Check sheet for the modelled part. Datum: model origin and axes. Units: mm. Round coordinates to 2 decimals unless told otherwise and drop trailing zeros. Loops run counter-clockwise (first coordinate to the right, second up) from the corner with the lowest first, then second, coordinate; pieces in that order, holes last. Notation, with made-up numbers: (5.5, 74) -> (42.5, 74) arc R19 cw to (42.5, 83) -> close; hole circle Ø2 at (71.5, 35). An arc over 180 degrees is marked (long way). Use one line per item in the form item = value. Start each with the question number.
(1) Sectioned sample at B-B (x = 4.75). Record the cut outline in (y, z), and give its area (3 significant figures).
(2) Material ranges on probe 1 along X at (y, z) = (40.5, -6.75); probe 2 along Y at (x, z) = (8.25, -12); probe 3 along X at (y, z) = (20, -13.5), recorded low to high. Write a range as [from, to].
(3) Sectioned sample at A-A (y = 13). Record the cut outline in (x, z).
from build123d import *

# Parameters (mm, degrees)
SKETCH1_W           = 15
SKETCH1_H           = 15
BOSS_EXTRUDE1_DEPTH = 120
CUT_EXTRUDE1_DEPTH  = 110
CUT_EXTRUDE2_START  = -20.25
CUT_EXTRUDE2_DEPTH  = 1.5
LPATTERN1_COUNT     = 27
LPATTERN1_PITCH     = 3
CUT_EXTRUDE3_START  = -10
SKETCH6_W           = 7
SKETCH6_H           = 7
CUT_EXTRUDE3_DEPTH  = 5.5


with BuildPart() as part:
    # Sketch1 → Boss-Extrude1 (new body)
    with BuildSketch(Plane(origin=(0, 0, 0), x_dir=(1, 0, 0), z_dir=(0, 1, 0))):
        with Locations((7.5, 7.5)):
            Rectangle(SKETCH1_W, SKETCH1_H)
    extrude(amount=BOSS_EXTRUDE1_DEPTH)

    # Sketch3 → Cut-Extrude1 (cut)
    with BuildSketch(Plane(origin=(0, 120, 0), x_dir=(1, 0, 0), z_dir=(0, 1, 0))):
        Polygon((15, 3), (13, 3), (13, 2), (11, 2), (11, 7.5), (13, 7.5), (13, 6.5), (15, 6.5), align=None)
        Polygon((3, 13), (2, 13), (2, 11), (7.5, 11), (7.5, 13), (6.5, 13), (6.5, 15), (3, 15), align=None)
    extrude(amount=-CUT_EXTRUDE1_DEPTH, mode=Mode.SUBTRACT)

    # Sketch5 → Cut-Extrude2 (cut)
    with BuildSketch(Plane(origin=(0, 120, 0), x_dir=(1, 0, 0), z_dir=(0, 1, 0)).offset(CUT_EXTRUDE2_START)):
        Polygon((15, 15), (15, 9.5), (9.5, 15), align=None)
    cut_extrude2 = extrude(amount=-CUT_EXTRUDE2_DEPTH, mode=Mode.SUBTRACT)

    # LPattern1: Cut-Extrude2 ×27
    with Locations(*[(0, -i * LPATTERN1_PITCH, 0) for i in range(1, LPATTERN1_COUNT)]):
        add(cut_extrude2, mode=Mode.SUBTRACT)

    # Sketch6 → Cut-Extrude3 (cut)
    with BuildSketch(Plane.XZ.offset(CUT_EXTRUDE3_START)):
        with Locations((11.5, -11.5)):
            Rectangle(SKETCH6_W, SKETCH6_H)
    extrude(amount=-CUT_EXTRUDE3_DEPTH, mode=Mode.SUBTRACT)


solid = part.part
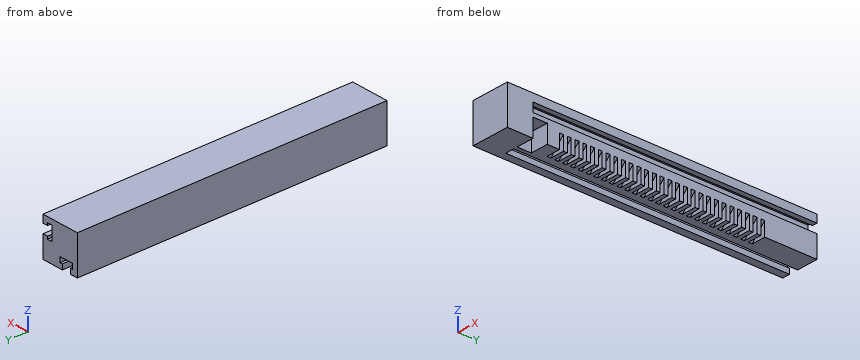
Checks:
q1.outline = (0, -15) -> (10, -15) -> (10, -11) -> (120, -11) -> (120, 0) -> (0, 0) -> close
q1.area = 1,360 mm2
q2.probe_1 = [0, 11], [13, 15]
q2.probe_2 = [0, 10], [15.5, 120]
q2.probe_3 = [0, 3], [6.5, 15]
q3.outline = (0, -15) -> (3, -15) -> (3, -13) -> (2, -13) -> (2, -11) -> (7.5, -11) -> (7.5, -13) -> (6.5, -13) -> (6.5, -15) -> (8, -15) -> (8, -8) -> (15, -8) -> (15, -6.5) -> (13, -6.5) -> (13, -7.5) -> (11, -7.5) -> (11, -2) -> (13, -2) -> (13, -3) -> (15, -3) -> (15, 0) -> (0, 0) -> close
